Autodesk Inventor part; units mm, degrees
ref_plane "YZ Plane" through (0, 0, 0) normal (1, 0, 0) x (0, 1, 0)
ref_plane "XZ Plane" through (0, 0, 0) normal (0, 1, 0) x (-1, 0, 0)
ref_plane "XY Plane" through (0, 0, 0) normal (0, 0, 1) x (1, 0, 0)
sketch "Sketch1" plane through (0, 0, 0) normal (0, 0, 1) x (1, 0, 0)
  line L0 (-21.2887, 16.8434) -> (23.7113, 16.8434)
  line L1 (23.7113, 16.8434) -> (23.7113, -34.1566)
  line L2 (23.7113, -34.1566) -> (-21.2887, -34.1566)
  line L3 (-21.2887, -34.1566) -> (-21.2887, 16.8434)
  point P0 (0, 0)
  dimension "d0" = 45
  dimension "d1" = 51
extrude "Extrusion1" add sketch "Sketch1" along normal blind 3.175
sketch "Sketch2" plane through (0, 0, 3.175) normal (0, 0, 1) x (1, 0, 0)
  line L0 (-21.2887, -34.1566) -> (-21.2887, 16.8434)
  line L1 (-21.2887, -34.1566) -> (-21.2887, -9.1566)
  circle A0 centre (-5.2887, -9.1566) radius 8
  circle A1 centre (-13.2887, -9.1566) radius 1
  circle A2 centre (-5.2887, -1.1566) radius 1
  circle A3 centre (2.7113, -9.1566) radius 1
  circle A4 centre (-5.2887, -17.1566) radius 1
  point P0 (0, 0)
  dimension "d4" = 25
  dimension "d6" = 16
  dimension "d7" = 2
  dimension "d8" = 2
  dimension "d9" = 2
  dimension "d10" = 2
  dimension "d11" = 16
extrude "Extrusion2" cut sketch "Sketch2" against normal blind 25.4 contours A0 A3 | A0 A3 | A2 A0 | A0 A2 | A4 A0 | A0 A4 | A1 A0 | A0 A1
sketch "Sketch3" plane through (0, 0, 3.175) normal (0, 0, 1) x (1, 0, 0)
  circle A0 centre (-5.2887, -9.1566) radius 1.9812
  point P0 (0, 0)
  dimension "d14" = 3.9624
extrude "Extrusion3" cut sketch "Sketch3" against normal blind 25.4
sketch "Sketch4" plane through (0, 0, 0) normal (0, 0, -1) x (-1, 0, 0)
  circle A0 centre (5.2887, -9.1566) radius 1.9812
  circle A1 centre (5.2887, -17.1566) radius 1
  circle A2 centre (13.2887, -9.1566) radius 1
  circle A3 centre (5.2887, -1.1566) radius 1
  circle A4 centre (-2.7113, -9.1566) radius 1
  line L0 (21.2887, 16.8434) -> (-23.7113, 16.8434)
  line L1 (-23.7113, 16.8434) -> (-23.7113, -34.1566)
  line L2 (-23.7113, -34.1566) -> (21.2887, -34.1566)
  line L3 (21.2887, -34.1566) -> (21.2887, 16.8434)
  line L4 (-23.7113, -34.1566) -> (-17.3613, -34.1566)
  point P0 (0, 0)
  dimension "d17" = 6.35
extrude "Extrusion4" add sketch "Sketch4" along normal blind 3.175
sketch "Sketch5" plane through (23.7113, -34.1566, 3.175) normal (1, 0, 0) x (0, 0, -1)
  line L0 (0, 51) -> (0, 0)
  line L1 (0, 0) -> (6.35, 0)
  line L2 (6.35, 0) -> (6.35, 51)
  line L3 (0, 51) -> (6.35, 51)
  point P0 (3.175, 34.1566)
extrude "Extrusion5" add sketch "Sketch5" along normal blind 3.175
properties part number "sidebase"
Here's how the part is built. I have some questions about the finished solid (model axes, mm). Coordinates: 2 decimals unless noted, no trailing zeros. Answer as a JSON object with one key per item and string values. Group by question number.
(1) If we mould it in two halves opening along X, with no side actions, what happens to faces 1 (the face through (-5.16, -7.18, 0.04)), 2 (the face through (8, -9, -3.175)), 3 (the face through (-21.289, -9, 0))? For each: released by +X, released by -X, zero draft, split by the parting line, or undercut.
(2) I need wall thicknesses on probe 1 along X at (y, z) = (-8.5, 2.75); probe 2 along X at (y, z) = (-10, 1.5); probe 3 along X at (y, z) = (-7.5, -0.5). Which ranges of each line are inside material? Lowest first, please.
(3) For pin 1 (1.6 mm diameter, centred on x = -13.29, y = -9.16, fed in from -Z), with a flat end and sliding along its axis, tell me the tip position at first contact or that it passes through.
Values found:
{
 "1": {"face 1": "undercut", "face 2": "zero draft", "face 3": "released by -X"},
 "2": {"probe 1": "x = -21.29 to -14.04, -12.53 to -7.16, -3.42 to 1.96, 3.47 to 26.89", "probe 2": "x = -21.29 to -13.83, -12.75 to -7.08, -3.5 to 2.17, 3.25 to 26.89", "probe 3": "x = -21.29 to -6.38, -4.2 to 26.89"},
 "3": {"pin 1": "passes through"}
}
